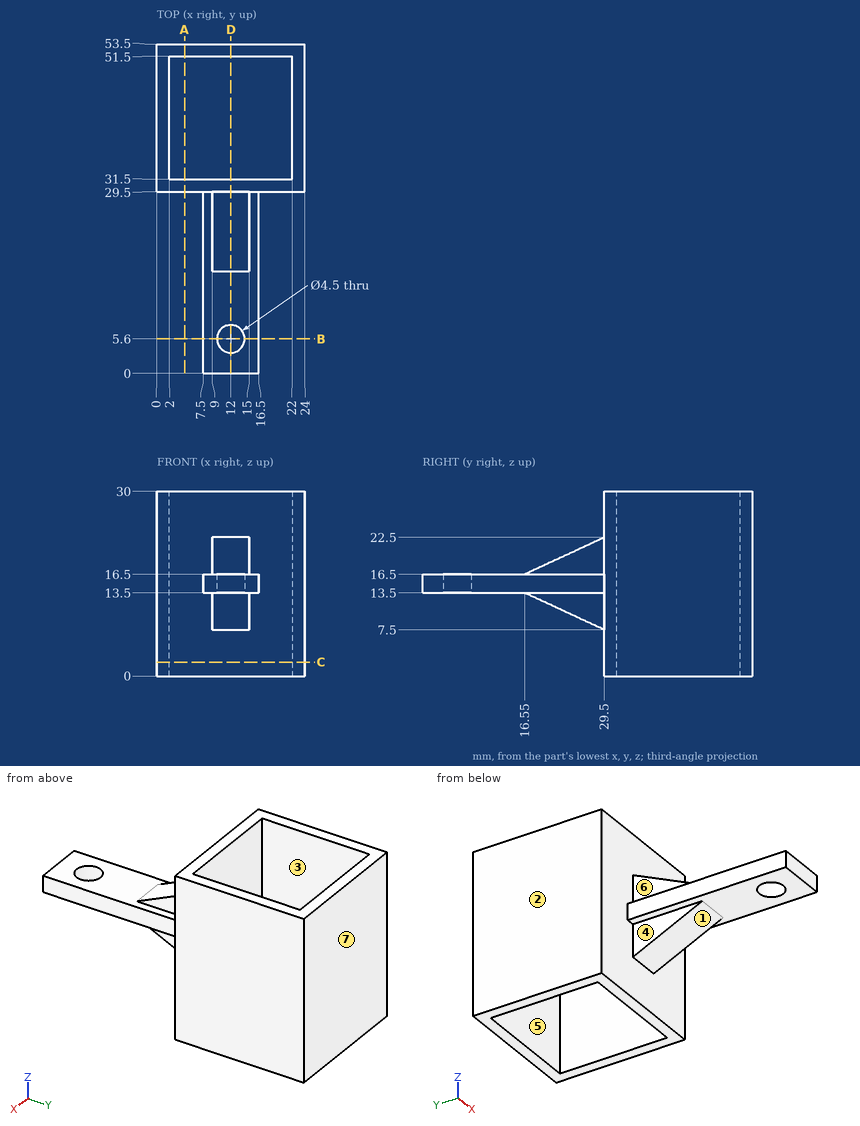
Study the drawing (mm; zero at the part's minimum x, y, z) and answer. A direction names the side the tool comes from. Round coordinates to 2 decimals unless told otherwise and drop trailing zeros. Write each loop counter-clockwise with the first axis right and the second up, starting at its lowest first coordinate (ties: lowest second). Pieces come first, ordered by that corner, then holes. Notation, with made-up numbers: (-29, -31) - (-1, -31) arc R19 cw to (-1, -20) - close; hole circle Ø8 at (76.25, 8). An arc over 180 degrees is marked (long way). Return JSON: item names as keys, results as strings. Group by question number.
Q1. Find the intervals of material crossed by L1, parallel to Y at x = 12, z = 15.5; L2, parallel to Y at x = 13.5, z = 28.5; L3, parallel to X at y = 46, z = 22.5, in increasing order.
Q2. The part is cut by section C-C on z = 2.25. Write down the section's boundary in (x, y), then the cut area to 3 significant figures.
Q3. For the marked faces 4, 5, 6 and 7, determine the directions among +Z, -Z, +X, -X, +Y, -Y from which every point of the face is accessible in a straight line to the end or side of a thin tool.
Q4. The mould has two halves that part along Y. Classify the marked faces 1, 2 and 3: released by +Y, released by -Y, zero draft, split by the parting line, or undercut.
Q5. Each of these flat-tipped pins is pushed along its axis until it touches: pin 1 Ø6.5 at (y, z) = (25, 20) entering from -X; pin 2 Ø7 at (x, y) = (13, 7.5) entering from -Z; pin 3 Ø5 at (y, z) = (22.5, 19.5) entering from +X. Where does it stop, or does it pass through?
Q6. The part is cut by section B-B on y = 5.6. Write down the section's boundary in (x, z).
Q7. The part is cut by section D-D on x = 12. Write down the section's boundary in (y, z).
Q8. The part is cut by section A-A on x = 4.5. Write down the section's boundary in (y, z), then the cut area to 3 significant figures.
Solved:
{
 "1": {"L1": "0 to 3.35, 7.85 to 31.5, 51.5 to 53.5", "L2": "29.5 to 31.5, 51.5 to 53.5", "L3": "0 to 2, 22 to 24"},
 "2": {"outline": "(0, 29.5) - (24, 29.5) - (24, 53.5) - (0, 53.5) - close; hole (2, 31.5) - (22, 31.5) - (22, 51.5) - (2, 51.5) - close", "area": "176 mm²"},
 "3": {"face 4": "-Z, -X, -Y", "face 5": "+Z, -Z", "face 6": "+Z, -X, -Y", "face 7": "+Z, -Z, +X, -X, +Y"},
 "4": {"face 1": "released by -Y", "face 2": "zero draft", "face 3": "undercut"},
 "5": {"pin 1": "x = 9", "pin 2": "z = 13.5", "pin 3": "x = 15"},
 "6": {"outline": "(7.5, 13.5) - (9.75, 13.5) - (9.75, 16.5) - (7.5, 16.5) - close; (14.25, 13.5) - (16.5, 13.5) - (16.5, 16.5) - (14.25, 16.5) - close"},
 "7": {"outline": "(0, 13.5) - (3.35, 13.5) - (3.35, 16.5) - (0, 16.5) - close; (7.85, 13.5) - (16.55, 13.5) - (29.5, 7.5) - (29.5, 0) - (31.5, 0) - (31.5, 30) - (29.5, 30) - (29.5, 22.5) - (16.55, 16.5) - (7.85, 16.5) - close; (51.5, 0) - (53.5, 0) - (53.5, 30) - (51.5, 30) - close"},
 "8": {"outline": "(29.5, 0) - (31.5, 0) - (31.5, 30) - (29.5, 30) - close; (51.5, 0) - (53.5, 0) - (53.5, 30) - (51.5, 30) - close", "area": "120 mm²"}
}
